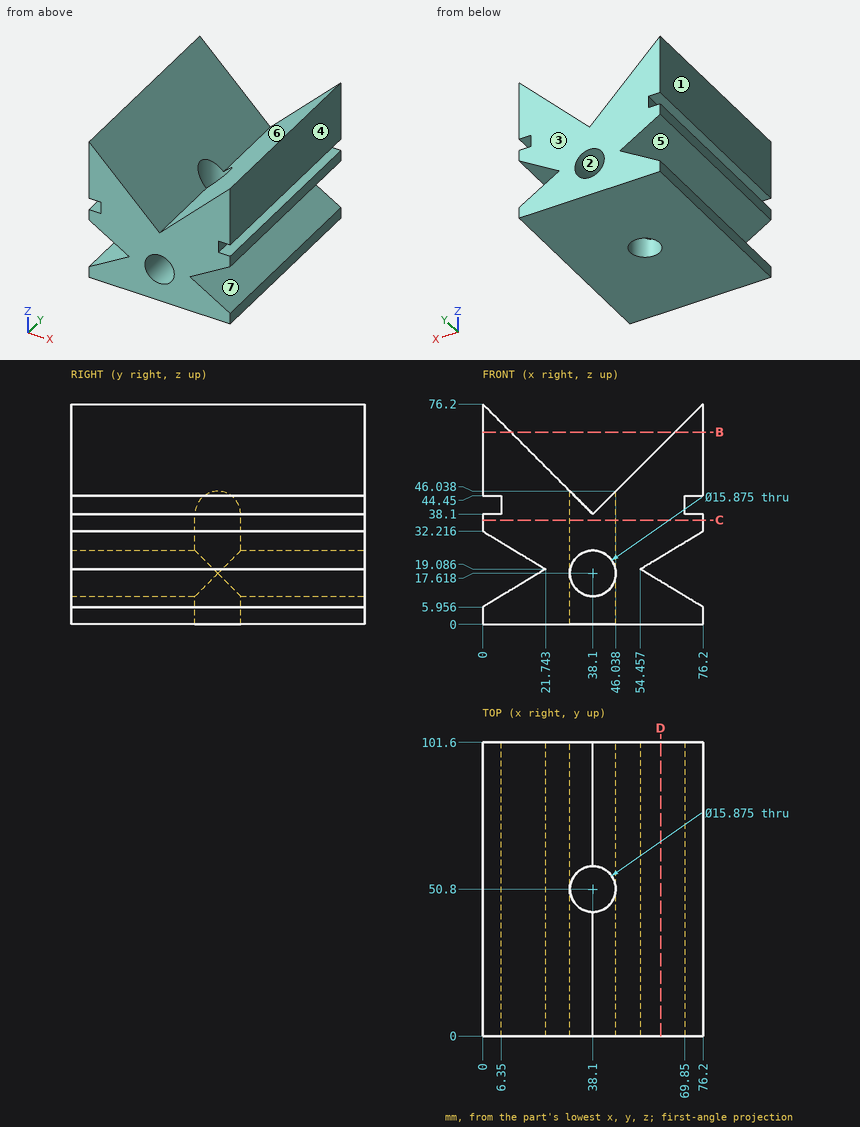
Input: dimensioned drawing with shaded views. Units: mm. Origin: part minimum x, y, z. A direction names the side the tool comes from. Coordinates: 2 decimals unless noted, no trailing zeros. Loops run counter-clockwise (first coordinate to the right, second up) from the corner with the lowest first, then second, coordinate; pieces in that order, holes last.
Q1. Section C-C, the plane z = 36. Return the cut outline in (x, y) (1 decimal).
Results are:
outline: (0, 0) - (76.2, 0) - (76.2, 101.6) - (0, 101.6) - close; hole circle Ø15.9 at (38.1, 50.8)
Q2. Section B-B, the plane z = 66.5. Return the cut outline in (x, y), and give its area (3 significant figures).
Results are:
outline: (0, 0) - (9.7, 0) - (9.7, 101.6) - (0, 101.6) - close; (66.5, 0) - (76.2, 0) - (76.2, 101.6) - (66.5, 101.6) - close
area: 1,970 mm2
Q3. Section D-D, the plane x = 61.5. Return the cut outline in (y, z), and give its area (3 significant figures).
Results are:
outline: (0, 0) - (101.6, 0) - (101.6, 14.83) - (0, 14.83) - close; (0, 23.34) - (101.6, 23.34) - (101.6, 61.5) - (0, 61.5) - close
area: 5,380 mm2
Q4. Set-up query: the marked faces 5, 6 and 7. Return all of +Z, -Z, +X, -X, +Y, -Y with unobstructed straight access to the full face (end or side cutting, diameter ignored); none if empty.
Results are:
face 5: -X, +Y, -Y
face 6: +Z, +Y, -Y
face 7: +X, +Y, -Y
Q5. Contact query for flat-ended pins moving along their axis: pin 1 (1.9 mm diameter, centred on y = 46, z = 42.5, fed in from -X); pin 2 (8 mm diameter, centred on x = 47.5, y = 84.5, fed in from +Z); pin 3 (18.5 mm diameter, centred on x = 38.1, y = 50.8, fed in from +Z). Output: stop coordinate, or through.
Results are:
pin 1: stops at x = 6.35
pin 2: stops at z = 51.5
pin 3: stops at z = 47.35
Q6. Line query: line 1 along Z through (x, y) = (38.1, 74.5) (1 decimal); line 2 along Y through (x, z) = (38.1, 30.75); line 3 along X through (y, z) = (95.5, 60.5). Output: solid intervals per line, ascending.
Results are:
line 1: z = 0 to 9.7, 25.6 to 38.1
line 2: y = 0 to 42.86, 58.74 to 101.6
line 3: x = 0 to 15.7, 60.5 to 76.2
Q7. Mould query, pull axis X, two halves, no side actions, for the marked faces 1, 2, 3 and 4. Classes: +X half, -X half, draft (parallel to the pull), parting line (faces both ways), or undercut.
Results are:
face 1: -X half
face 2: undercut
face 3: draft
face 4: +X half
